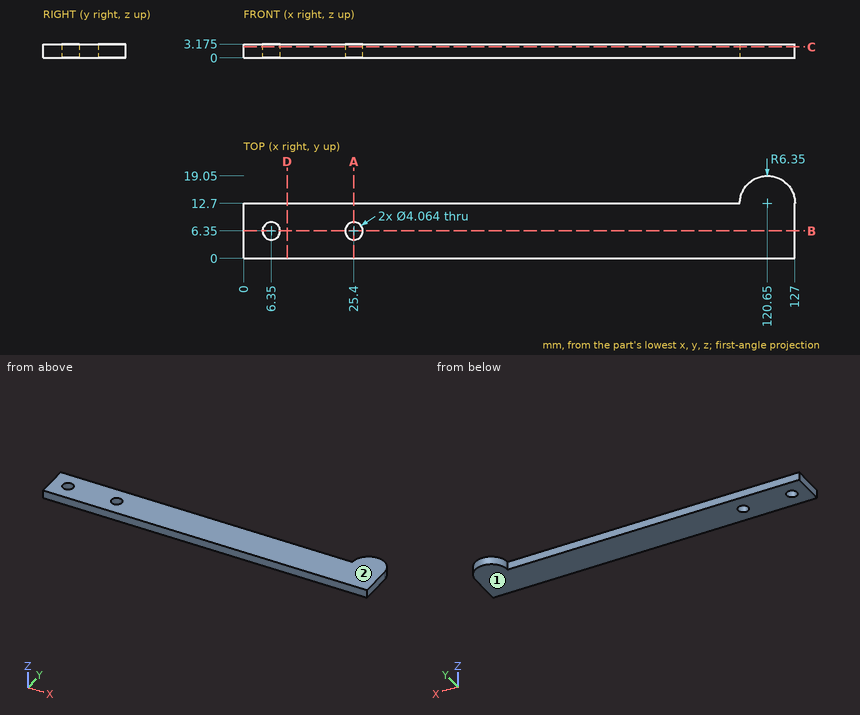
Answer from the drawing. Dimensions are ordinates in mm from the lowest x, y and z of the part. Round coordinates to 2 decimals unless told otherwise and drop trailing zeros. Loops run counter-clockwise (first coordinate to the right, second up) from the corner with the lowest first, then second, coordinate; pieces in that order, holes last. Notation, with made-up numbers: M -20.75,35.25 L 22.25,35.25 A35 cw 22.25,74.25 Z; hole C 73.25,-22.5 d1. An arc over 180 degrees is marked long. One line per question, with ' | ' between items. Start each with the question number.
(1) A cutting plane is placed at A-A on x = 25.4. Write down the section's boundary in (y, z) (3 decimals).
(2) A flat-ended cylindrical pin translates along its axis: pin 1 Ø1 at (x, z) = (34, 2) entering from +Y. Find the tip coordinate at first contact, or state that the pin passes through.
(3) A cutting plane is placed at D-D on x = 10. Write down the section's boundary in (y, z) (3 decimals).
(4) A cutting plane is placed at B-B on y = 6.35. Write down the section's boundary in (x, z) (3 decimals), plus the area to 3 significant figures.
(5) Find the intervals of material crossed by line 1 (X direction, y = 6, z = 2.2); line 2 (X direction, y = 5.75, z = 0.55); line 3 (Y direction, x = 6.35, z = 2.45), in increasing order.
(6) For a pull along Z with two mould halves and no side action, classify the marked faces 1 and 2 as released by +Z, released by -Z, zero draft, split by the parting line, or undercut.
(7) A cutting plane is placed at C-C on z = 2.5. Write down the section's boundary in (x, y).
Geometry check:
1) outline: M 0,0 L 4.318,0 L 4.318,3.175 L 0,3.175 Z; M 8.382,0 L 12.7,0 L 12.7,3.175 L 8.382,3.175 Z
2) pin 1: stops at y = 12.7
3) outline: M 0,0 L 12.7,0 L 12.7,3.175 L 0,3.175 Z
4) outline: M 0,0 L 4.318,0 L 4.318,3.175 L 0,3.175 Z; M 8.382,0 L 23.368,0 L 23.368,3.175 L 8.382,3.175 Z; M 27.432,0 L 127,0 L 127,3.175 L 27.432,3.175 Z | area: 377 mm²
5) line 1: x = 0 to 4.35, 8.35 to 23.4, 27.4 to 127 | line 2: x = 0 to 4.41, 8.29 to 23.46, 27.34 to 127 | line 3: y = 0 to 4.32, 8.38 to 12.7
6) face 1: released by -Z | face 2: released by +Z
7) outline: M 0,0 L 127,0 L 127,12.7 A6.35 ccw 114.3,12.7 L 0,12.7 Z; hole C 6.35,6.35 d4.06; hole C 25.4,6.35 d4.06
